The drawing under review shows one solid part. Ordinate dimensions are in mm from its lowest x, y, z. Round coordinates to 2 decimals unless told otherwise and drop trailing zeros. Write each loop counter-clockwise with the first axis right and the second up, starting at its lowest first coordinate (ties: lowest second). Pieces come first, ordered by that corner, then holes. Notation, with made-up numbers: (79, 85) - (96, 85) arc R13 cw to (96, 110) - close; hole circle Ø5 at (-35, 81.5). An arc over 180 degrees is marked (long way). Answer in a Markdown table with one row per item. Add a question column.
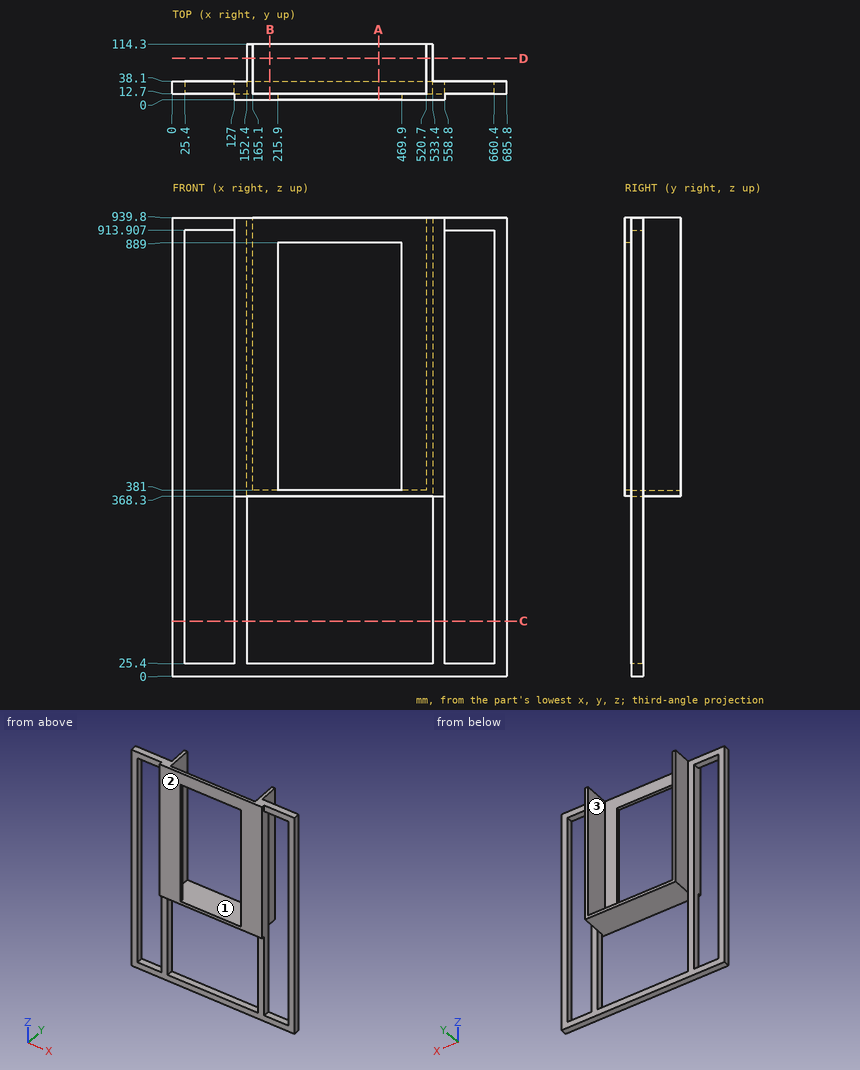
Q1. Add section C-C on z = 112.5. State the section outline as (x, y) points, then the cut area to 3 significant figures.
Q2. To check wall thickness, follow probe 1 along Z at (x, y) = (392.5, 26); probe 2 along X at (y, z) = (15, 876.5); probe 3 along X at (y, z) = (87, 642.5). State the ranges of each line that lie inside material, in increasing order.
Q3. Add section D-D on y = 85. State the section outline as (x, z) points.
Q4. Insertion check: pin 1 Ø1 at (x, y) = (399.5, 47.5) entering from +Z; pin 2 Ø23 at (y, z) = (67, 532.5) entering from -X; pin 3 Ø2 at (x, y) = (423, 66) entering from -Z. Each pin has a flat end and moves straight along its axis. Give the tip position at first contact, or say it passes through.
Q5. Draft analysis for pull direction X (two halves, no side actions). For the marked faces 1, 2 and 3, state which applies: released by +X, released by -X, zero draft, split by the parting line, or undercut.
Q6. Add section A-A on x = 423. State the section outline as (y, z) points, then the cut area to 3 significant figures.
Q7. Add section B-B on x = 200. State the section outline as (y, z) points.
Answer sheet:
| question | item | result |
|---|---|---|
| 1 | outline | (0, 12.7) - (25.4, 12.7) - (25.4, 38.1) - (0, 38.1) - close; (127, 12.7) - (152.4, 12.7) - (152.4, 38.1) - (127, 38.1) - close; (533.4, 12.7) - (558.8, 12.7) - (558.8, 38.1) - (533.4, 38.1) - close; (660.4, 12.7) - (685.8, 12.7) - (685.8, 38.1) - (660.4, 38.1) - close |
| 1 | area | 2,580 mm² |
| 2 | probe 1 | z = 0 to 25.4, 368.3 to 381 |
| 2 | probe 2 | x = 0 to 25.4, 127 to 165.1, 520.7 to 558.8, 660.4 to 685.8 |
| 2 | probe 3 | x = 152.4 to 165.1, 520.7 to 533.4 |
| 3 | outline | (152.4, 368.3) - (533.4, 368.3) - (533.4, 939.8) - (520.7, 939.8) - (520.7, 381) - (165.1, 381) - (165.1, 939.8) - (152.4, 939.8) - close |
| 4 | pin 1 | stops at z = 381 |
| 4 | pin 2 | stops at x = 152.4 |
| 4 | pin 3 | stops at z = 368.3 |
| 5 | face 1 | undercut |
| 5 | face 2 | zero draft |
| 5 | face 3 | undercut |
| 6 | outline | (0, 368.3) - (114.3, 368.3) - (114.3, 381) - (0, 381) - close; (0, 889) - (12.7, 889) - (12.7, 939.8) - (0, 939.8) - close; (12.7, 0) - (38.1, 0) - (38.1, 25.4) - (12.7, 25.4) - close |
| 6 | area | 2,740 mm² |
| 7 | outline | (0, 368.3) - (114.3, 368.3) - (114.3, 381) - (12.7, 381) - (12.7, 939.8) - (0, 939.8) - close; (12.7, 0) - (38.1, 0) - (38.1, 25.4) - (12.7, 25.4) - close |
